```python
from build123d import *

# Parameters (mm, degrees)
SKETCH1_R           = 6
SKETCH1_R_2         = 2
BOSS_EXTRUDE1_DEPTH = 4
CUT_EXTRUDE2_DEPTH  = 5
CIRPATTERN2_COUNT   = 10
SKETCH11_R          = 4
BOSS_EXTRUDE2_DEPTH = 11
CUT_EXTRUDE3_START  = 11
CUT_EXTRUDE3_DEPTH  = 2
CUT_EXTRUDE4_DEPTH  = 12


with BuildPart() as part:
    # Sketch1 → Boss-Extrude1 (new body)
    with BuildSketch(Plane.XY):
        Circle(SKETCH1_R)
        Circle(SKETCH1_R_2, mode=Mode.SUBTRACT)
    extrude(amount=BOSS_EXTRUDE1_DEPTH)

    # Sketch4 → Cut-Extrude2 (cut, through all)
    with BuildSketch(Plane.XY):
        with BuildLine():
            ThreePointArc((-0.50024657, 3.968595894), (0, 4), (0.50024657, 3.968595894))
            ThreePointArc((0.50024657, 3.968595894), (1.074726656, 5.403066604), (2.5, 6))
            ThreePointArc((2.5, 6), (0, 6.5), (-2.5, 6))
            ThreePointArc((-2.5, 6), (-1.085786438, 5.414213562), (-0.5, 4))
            ThreePointArc((-0.5, 4), (-0.500061643, 3.984297463), (-0.50024657, 3.968595894))
        make_face()
    cut_extrude2 = extrude(amount=CUT_EXTRUDE2_DEPTH, mode=Mode.SUBTRACT)

    # CirPattern2: Cut-Extrude2 ×10 about axis
    cirpattern2_axis = Axis((0, 0, 0), (0, 0, 1))
    for i in range(1, CIRPATTERN2_COUNT):
        add(cut_extrude2.rotate(cirpattern2_axis, i * 360 / CIRPATTERN2_COUNT), mode=Mode.SUBTRACT)

    # Sketch11 → Boss-Extrude2 (add)
    with BuildSketch(Plane.XY):
        Circle(SKETCH11_R)
    extrude(amount=BOSS_EXTRUDE2_DEPTH)

    # Sketch12 → Cut-Extrude3 (cut)
    with BuildSketch(Plane.XY.offset(CUT_EXTRUDE3_START)):
        Polygon((3.290896534, 0), (1.645448267, 2.85), (-1.645448267, 2.85), (-3.290896534, 0), (-1.645448267, -2.85), (1.645448267, -2.85), align=None)
    extrude(amount=-CUT_EXTRUDE3_DEPTH, mode=Mode.SUBTRACT)

    # Sketch13 → Cut-Extrude4 (cut, through all)
    with BuildSketch(Plane.XY):
        with BuildLine():
            Line((1.6, 0.95), (-1.6, 0.95))
            ThreePointArc((-1.6, 0.95), (0, -1.860779407), (1.6, 0.95))
        make_face()
    extrude(amount=CUT_EXTRUDE4_DEPTH, mode=Mode.SUBTRACT)


solid = part.part
```
Check sheet for the modelled part. Datum: model origin and axes. Units: mm. A direction names the side the tool comes from. Coordinates: 2 decimals unless noted, no trailing zeros. Order: outer loops, then holes, each group sorted by start corner. A loop starts at its lowest first (then second) coordinate and runs counter-clockwise, first axis right, second up. Notation, with made-up numbers: (77, 82) -> (102, 82) arc R33 cw to (102, 120) -> close; hole circle Ø1 at (19.25, -14.75). An arc over 180 degrees is marked (long way). Write each question's results on one line, items separated by ' | '. Start each with the question number.
1) Material ranges on line 1 along Y through (x, z) = (0, 4.5); line 2 along X through (y, z) = (0, 4.5); line 3 along Z through (x, y) = (-4.25, 3), recorded low to high.
2) Section check B-B (x = 0). Enter the section's corners in (y, z).
3) Set-up check for faces 4 (the face through (-4, -3, 4)), 5 (the face through (4, -3, 4)), 6 (the face through (0, 1.3, 9)): record each of +Z, -Z, +X, -X, +Y, -Y from which the full face is reachable in a straight line by a thin tool's end or side.
4) Depth check by flat-ended pin: pin 1 (2 mm diameter, centred on x = 0.5, z = 9.5, fed in from -Y); pin 2 (1.6 mm diameter, centred on x = -1, z = 10, fed in from +Y) (3 decimals); pin 3 (3 mm diameter, centred on x = 4, y = 3, fed in from +Z); pin 4 (1 mm diameter, centred on y = -4, z = 2.5, fed in from +X). Enter the tip coordinate at first touch or a pass-through.
5) Draft check along X on faces 1 (the face through (-1, -5, 4)), 2 (the face through (-3.581, -3.603, 1.972)), 3 (the face through (-4.564, -2.328, 1.972)). Enter one of: pulls with the +X half, pulls with the -X half, needs draft (parallel to the pull), parting line crosses it, or undercut.
6) Section check D-D (y = 2). Enter the section's corners in (x, z), and give its area (3 significant figures).
7) Section check C-C (y = 5.25). Enter the section's corners in (x, z).
8) Section check A-A (z = 9.25). Enter the section's corners in (x, y), and give its area (3 significant figures).
Checked values:
1) line 1: -4 to -1.86, 0.95 to 4 | line 2: -4 to -1.86, 1.86 to 4 | line 3: 0 to 4
2) outline: (-4, 0) -> (-1.86, 0) -> (-1.86, 9) -> (-2.85, 9) -> (-2.85, 11) -> (-4, 11) -> close; (0.95, 0) -> (4, 0) -> (4, 11) -> (2.85, 11) -> (2.85, 9) -> (0.95, 9) -> close
3) face 4: +Z, -X, -Y | face 5: +Z, +X, -Y | face 6: +Z
4) pin 1: y = -4 | pin 2: y = 3.995 | pin 3: z = 11 | pin 4: x = 4.87
5) face 1: needs draft | face 2: undercut | face 3: pulls with the -X half
6) outline: (-4.21, 0) -> (4.21, 0) -> (4.21, 4) -> (3.46, 4) -> (3.46, 11) -> (2.14, 11) -> (2.14, 9) -> (-2.14, 9) -> (-2.14, 11) -> (-3.46, 11) -> (-3.46, 4) -> (-4.21, 4) -> close | area: 73.7 mm²
7) outline: (-2.25, 0) -> (-0.94, 0) -> (-0.94, 4) -> (-2.25, 4) -> close; (0.94, 0) -> (2.25, 0) -> (2.25, 4) -> (0.94, 4) -> close
8) outline: circle Ø8 at (0, 0); hole (-3.29, 0) -> (-1.65, -2.85) -> (1.65, -2.85) -> (3.29, 0) -> (1.65, 2.85) -> (-1.65, 2.85) -> close | area: 22.1 mm²
